```python
from build123d import *

# Parameters (mm, degrees)
SKETCH1_W                = 20
SKETCH1_H                = 6
BOSS_EXTRUDE1_DEPTH      = 13
CUT_EXTRUDE1_REACH       = 51.362
SKETCH2_R                = 2.6
BOSS_EXTRUDE2_DEPTH      = 3
BOSS_EXTRUDE2_DEPTH_BACK = 3
SKETCH3_W                = 13
SKETCH3_H                = 20
SKETCH4_R                = 1.025
CUT_EXTRUDE2_DEPTH       = 5.9
FILLET1_R                = 1
FILLET2_R                = 1


with BuildPart() as part:
    # Sketch1 → Boss-Extrude1 (new body)
    with BuildSketch(Plane(origin=(32.364284334, 0, 0), x_dir=(0, 0, -1), z_dir=(1, 0, 0))):
        with Locations((-7.875866483, 38.765059464)):
            Rectangle(SKETCH1_W, SKETCH1_H)
        with BuildLine():
            Line((-12.22448084, 35.533673821), (-10.765866483, 34.075059464))
            Line((-10.765866483, 34.075059464), (-4.985866483, 34.075059464))
            Line((-4.985866483, 34.075059464), (-3.527252126, 35.533673821))
            ThreePointArc((-3.527252126, 35.533673821), (-3.27095768, 35.704924294), (-2.968637768, 35.765059464))
            Line((-2.968637768, 35.765059464), (-12.783095197, 35.765059464))
            ThreePointArc((-12.783095197, 35.765059464), (-12.480775285, 35.704924294), (-12.22448084, 35.533673821))
        make_face()
    extrude(amount=BOSS_EXTRUDE1_DEPTH)

    # Sketch2 → Cut-Extrude1 (cut, up to next)
    with BuildSketch(Plane.XZ.offset(-34.075059464), mode=Mode.PRIVATE) as cut_extrude1_sk1:
        with Locations(Location((38.864284334, 7.875866483, 0), (0, 0, 270))):
            Circle(SKETCH2_R)
    cut_extrude1_tool1 = extrude(cut_extrude1_sk1.sketch, amount=-CUT_EXTRUDE1_REACH, mode=Mode.PRIVATE) & part.part
    add(cut_extrude1_tool1.solids().sort_by_distance((38.864284, 34.075059, 7.875866))[0], mode=Mode.SUBTRACT)

    # Sketch3 → Boss-Extrude2 (add, two sides: drawn at the far end of the back side and taken through both)
    with BuildSketch(Plane.XY.offset(17.875866483).offset(-BOSS_EXTRUDE2_DEPTH_BACK)):
        with Locations((38.864284334, 45.765059464)):
            Rectangle(SKETCH3_W, SKETCH3_H)
    extrude(amount=BOSS_EXTRUDE2_DEPTH + BOSS_EXTRUDE2_DEPTH_BACK)

    # Sketch4 → Cut-Extrude2 (cut)
    with BuildSketch(Plane.XY.offset(20.875866483)):
        with Locations((38.364284334, 50.565059464)):
            Circle(SKETCH4_R)
        with Locations((38.364284334, 40.965059464)):
            Circle(SKETCH4_R)
    extrude(amount=-CUT_EXTRUDE2_DEPTH, mode=Mode.SUBTRACT)

    # Fillet1
    # the kernel refuses this fillet: 1 mm, written as the material it adds along each edge
    with BuildSketch(Plane(origin=(45.364284334, 41.765059464, 14.875866483), x_dir=(0, 0, -1), z_dir=(-1, 0, 0))) as fillet1_piece_1:
        with BuildLine():
            CenterArc((FILLET1_R, -FILLET1_R), FILLET1_R, 90, 90)
            Line((0, -FILLET1_R), (0, 0))
            Line((0, 0), (FILLET1_R, 0))
        make_face()
    extrude(amount=13)
    # the kernel refuses this fillet: 1 mm, written as the material it takes off along each edge
    with BuildSketch(Plane(origin=(47.864284334, 55.765059464, 14.875866483), x_dir=(0, -1, 0), z_dir=(-1, 0, 0)), Plane(origin=(29.864284334, 35.765059464, 20.875866483), x_dir=(0, 0, -1), z_dir=(1, 0, 0))) as fillet1_2_piece_1:
        with BuildLine():
            CenterArc((FILLET1_R, FILLET1_R), FILLET1_R, 180, 90)
            Line((0, FILLET1_R), (0, 0))
            Line((0, 0), (FILLET1_R, 0))
        make_face()
    extrude(amount=18, mode=Mode.SUBTRACT)
    with BuildSketch(Plane(origin=(47.864284334, 55.765059464, 20.875866483), x_dir=(0, -1, 0), z_dir=(-1, 0, 0)), Plane(origin=(29.864284334, 41.765059464, -2.124133517), x_dir=(0, -1, 0), z_dir=(1, 0, 0)), Plane(origin=(29.864284334, 35.765059464, -2.124133517), x_dir=(0, 0, 1), z_dir=(1, 0, 0))) as fillet1_2_piece_2:
        with BuildLine():
            CenterArc((FILLET1_R, -FILLET1_R), FILLET1_R, 90, 90)
            Line((0, -FILLET1_R), (0, 0))
            Line((0, 0), (FILLET1_R, 0))
        make_face()
    extrude(amount=18, mode=Mode.SUBTRACT)
    with BuildSketch(Plane(origin=(31.328750428, 34.075059464, 4.985866483), x_dir=(0, 0, 1), z_dir=(1, 0, 0)), Plane(origin=(31.328750428, 34.075059464, 10.765866483), x_dir=(0, 0.7071067811865432, 0.7071067811865518), z_dir=(1, 0, 0))) as fillet1_2_piece_3:
        with BuildLine():
            CenterArc((FILLET1_R * 0.414213562373, -FILLET1_R), FILLET1_R, 90, 45)
            Line((-FILLET1_R * 0.292893218813, -FILLET1_R * 0.292893218813), (0, 0))
            Line((0, 0), (FILLET1_R * 0.414213562373, 0))
        make_face()
    extrude(amount=15.071067812, mode=Mode.SUBTRACT)

    # Fillet2
    fillet2_edges = [part.edges().sort_by_distance(p)[0] for p in [
        (45.364284334, 35.704924294, 12.480775285),
        (32.364284334, 35.765059464, 0.922252126),
        (32.364284334, 35.704924294, 3.27095768),
        (32.364284334, 34.950813252, 4.110112695),
        (32.364284334, 35.704924294, 12.480775285),
        (32.364284334, 48.765059464, 14.875866483),
        (32.364284334, 41.765059464, 6.375866483),
        (32.364284334, 38.765059464, -2.124133517),
        (32.364284334, 34.075059464, 7.875866483),
        (32.364284334, 34.950813252, 11.641620271),
        (32.364284334, 35.765059464, 16.32948084),
        (32.364284334, 45.765059464, 20.875866483),
        (32.364284334, 55.765059464, 17.875866483),
        (32.364284334, 36.057952683, 20.582973264),
        (32.364284334, 55.472166245, 15.168759702),
        (32.364284334, 41.472166245, -1.831240298),
        (32.364284334, 55.472166245, 20.582973264),
        (32.364284334, 36.057952683, -1.831240298),
        (32.364284334, 34.151179931, 10.734336353),
        (32.364284334, 34.151179931, 5.017396613),
        (45.364284334, 34.075059464, 7.875866483),
        (45.364284334, 41.765059464, 6.375866483),
        (45.364284334, 48.765059464, 14.875866483),
        (45.364284334, 55.765059464, 17.875866483),
        (45.364284334, 45.765059464, 20.875866483),
        (45.364284334, 35.765059464, 16.32948084),
        (45.364284334, 34.950813252, 11.641620271),
        (45.364284334, 38.765059464, -2.124133517),
        (45.364284334, 36.057952683, 20.582973264),
        (45.364284334, 55.472166245, 15.168759702),
        (45.364284334, 41.472166245, -1.831240298),
        (45.364284334, 55.472166245, 20.582973264),
        (45.364284334, 36.057952683, -1.831240298),
        (45.364284334, 34.151179931, 10.734336353),
        (45.364284334, 34.151179931, 5.017396613),
        (32.364284334, 42.057952683, 14.582973264),
        (45.364284334, 42.057952683, 14.582973264),
        (45.364284334, 34.950813252, 4.110112695),
        (45.364284334, 35.704924294, 3.27095768),
        (45.364284334, 35.765059464, 0.922252126),
    ]]
    fillet(fillet2_edges, radius=FILLET2_R)


solid = part.part
```
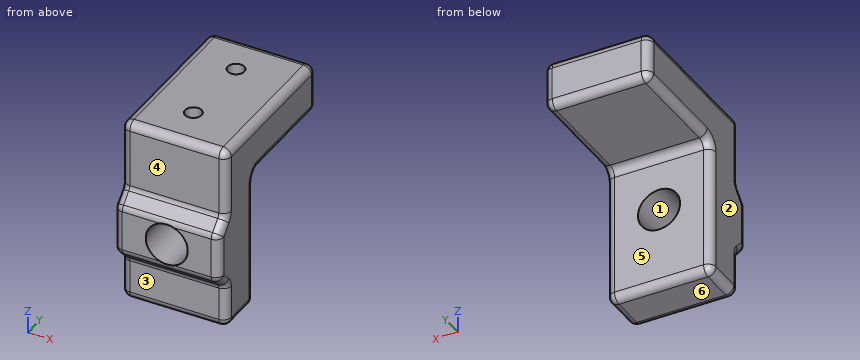
CAD build for the part. Positions are in the model's coordinates, mm. Face numbers are marked on the shaded views. A direction names the side the tool comes from. Coordinates: 2 decimals unless noted, no trailing zeros. Order: outer loops, then holes, each group sorted by start corner. A loop starts at its lowest first (then second) coordinate and runs counter-clockwise, first axis right, second up. Notation, with made-up numbers: (35, -16) -> (60, -16) arc R11 ccw to (60, -3) -> close; hole circle Ø6 at (41, -29.75). An arc over 180 degrees is marked (long way). Use one line per item in the form item = value. Start each with the question number.
1) Drop flat-ended pins along their axis: pin 1 (1.5 mm diameter, centred on x = 41, z = 4.5, fed in from +Y); pin 2 (0.6 mm diameter, centred on x = 38.5, y = 51, fed in from +Z); pin 3 (4 mm diameter, centred on x = 38.86, z = 7.88, fed in from +Y); pin 4 (2 mm diameter, centred on x = 39, z = 16.5, fed in from -Y). Give the stop position or say it passes through.
2) Pull direction X, two halves, no side cores. Call the marked faces 1, 2 and 3: +X half, -X half, draft (parallel to the pull), parting line (faces both ways), or undercut.
3) Tool access for the marked faces 4, 5 and 6: list every direction of +Z, -Z, +X, -X, +Y, -Y with a clear straight run to the whole face (end or side of a thin tool).
4) Band-saw the part on B-B on x = 41. Give the cut face in (y, z).
5) Band-saw the part on C-C on z = 1. Give the cut face in (x, y), then the cut area to 3 significant figures.
6) Band-saw the part on A-A on z = 9.5. Give the cut face in (x, y), then the cut area to 3 significant figures.
7) Band-saw the part on D-D on y = 54.25. Give the cut face in (x, z).
8) Drill centre lines: L1, parallel to Z at x = 41.25, y = 54.75; L2, parallel to Y at x = 34, z = -0.25; L3, parallel to Y at x = 34.25, z = 9. Where is each one in solid material? Low to high. Write a range as [from, to].
Entries:
q1.pin_1 = 41.77
q1.pin_2 = 14.98
q1.pin_3 = through
q1.pin_4 = 35.77
q2.face_1 = undercut
q2.face_2 = -X half
q2.face_3 = draft
q3.face_4 = +Z, +X, -X, -Y
q3.face_5 = -Z, +X, -X, +Y
q3.face_6 = -Z, +X, -X, +Y, -Y
q4.outline = (34.08, 5.4) arc R1 ccw to (34.37, 4.69) -> (35.53, 3.53) arc R0.79 cw to (35.77, 2.97) -> (35.77, -1.12) arc R1 ccw to (36.77, -2.12) -> (40.77, -2.12) arc R1 ccw to (41.77, -1.12) -> (41.77, 6.39) -> (34.08, 6.39) -> close; (34.08, 9.36) -> (41.77, 9.36) -> (41.77, 13.88) arc R1 cw to (42.77, 14.88) -> (54.77, 14.88) arc R1 ccw to (55.77, 15.88) -> (55.77, 19.88) arc R1 ccw to (54.77, 20.88) -> (36.77, 20.88) arc R1 ccw to (35.77, 19.88) -> (35.77, 12.78) arc R0.79 cw to (35.53, 12.22) -> (34.37, 11.06) arc R1 ccw to (34.08, 10.35) -> close
q5.outline = (32.36, 36.77) arc R1 ccw to (33.36, 35.77) -> (44.36, 35.77) arc R1 ccw to (45.36, 36.77) -> (45.36, 40.77) arc R1 ccw to (44.36, 41.77) -> (33.36, 41.77) arc R1 ccw to (32.36, 40.77) -> close
q5.area = 77.1 mm2
q6.outline = (32.36, 35.08) arc R1 ccw to (33.36, 34.08) -> (36.83, 34.08) -> (36.83, 41.77) -> (33.36, 41.77) arc R1 ccw to (32.36, 40.77) -> close; (40.89, 34.08) -> (44.36, 34.08) arc R1 ccw to (45.36, 35.08) -> (45.36, 40.77) arc R1 ccw to (44.36, 41.77) -> (40.89, 41.77) -> close
q6.area = 67.9 mm2
q7.outline = (32.36, 15.88) arc R1 ccw to (33.36, 14.88) -> (44.36, 14.88) arc R1 ccw to (45.36, 15.88) -> (45.36, 19.88) arc R1 ccw to (44.36, 20.88) -> (33.36, 20.88) arc R1 ccw to (32.36, 19.88) -> close
q8.L1 = [14.88, 20.88]
q8.L2 = [35.77, 41.77]
q8.L3 = [34.08, 41.77]
